Model file for the job. Use its own axes, mm. A direction names the side the tool comes from. Coordinates: 2 decimals unless noted, no trailing zeros. Order: outer loops, then holes, each group sorted by start corner. A loop starts at its lowest first (then second) coordinate and runs counter-clockwise, first axis right, second up. Notation, with made-up numbers: (-6.5, 30) -> (14.5, 30) arc R26 ccw to (14.5, 58) -> close; hole circle Ø3 at (-18, 80.25). An arc over 180 degrees is marked (long way). Return JSON: item names as keys, results as strings. Group by question number.
1) Pull direction Z, two halves, no side cores. Call faces 4 (the flat face through (-35, 2, 60)), 5 (the flat face through (-67.3, 118, 45.5)), 6 (the flat face through (-74, 121, 5)): +Z half, -Z half, draft (parallel to the pull), parting line (faces both ways), or undercut.
2) Cut at B-B (x = 58). Write the cut outline in (y, z), and give its area (3 significant figures).
3) Probe line 1 (Y direction, x = -75, z = -40); line 2 (X direction, y = 2.2, z = -52); line 3 (Y direction, x = -74.6, z = 12.5). List the from-to ranges inside material, lowest first.
4) Flat gauge pins, fed straight in: pin 1 (3.5 mm diameter, centred on x = -66, z = 46.9, fed in from +Y); pin 2 (10 mm diameter, centred on y = 49.5, z = -43.5, fed in from +X); pin 3 (2 mm diameter, centred on y = 117, z = 47.5, fed in from +X). Where does each tip first touch, or does it go through?
5) Cut at A-A (y = 113). Write the cut outline in (x, z), and give its area (3 significant figures).
6) Which spindle directions (+Z, -Z, +X, -X, +Y, -Y) get a long thin tool onto all of the face, cutting with end or side? Do faces 1 (the flat face through (-72, 67, 56.9)), 2 (the flat face through (-66, 116, 1)), 3 (the flat face through (-74, 57.418, 0)). Say none if no direction does.
from build123d import *

# Parameters (mm, degrees)
SKETCH1_W              = 154
SKETCH1_H              = 120
LARGE_WALL_OUTER_DEPTH = 3
SKETCH8_W              = 3
SKETCH8_H              = 120
SMALL_WALL_OUTER_DEPTH = 120.1
SKETCH10_W             = 113.8
SKETCH10_H             = 112.9
SMALL_WALL_INNER_DEPTH = 3
SKETCH14_W             = 113.8
SKETCH14_H             = 4
MOUNT_DEPTH            = 10
MOUNTING_NUTS_DEPTH    = 2
NUT_1_BOLT_HOLE_REACH  = 155.144
SKETCH18_R             = 1.5
NUT_2_BOLT_HOLE_REACH  = 155.144
SKETCH19_R             = 1.5
CONNECTOR_SLOTS_REACH  = 208.082
SKETCH23_R             = 1.5
SKETCH27_R             = 1.55
SKETCH27_R_2           = 1.5
PCB_MOUNT_HOLES_DEPTH  = 6
SKETCH28_R             = 1.5
BOLT_HOLE1_DEPTH       = 10
SKETCH29_R             = 1.5
BOLT_HOLE2_DEPTH       = 10
SKETCH30_R             = 1.5
BOLT_HOLES34_DEPTH     = 10


with BuildPart() as part:
    # Sketch1 → Large-Wall-Outer (new body)
    with BuildSketch(Plane(origin=(0, 0, 0), x_dir=(1, 0, 0), z_dir=(0, 1, 0))):
        Rectangle(SKETCH1_W, SKETCH1_H)
    extrude(amount=LARGE_WALL_OUTER_DEPTH)

    # Sketch8 → Small-Wall-Outer (add)
    with BuildSketch(Plane(origin=(0, 3, 0), x_dir=(1, 0, 0), z_dir=(0, 1, 0))):
        with Locations((-75.5, 0)):
            Rectangle(SKETCH8_W, SKETCH8_H)
    extrude(amount=SMALL_WALL_OUTER_DEPTH)

    # Sketch10 → Small-Wall-Inner (add)
    with BuildSketch(Plane(origin=(-74, 0, 0), x_dir=(0, 0, -1), z_dir=(1, 0, 0))):
        with Locations((0, 63.55)):
            Rectangle(SKETCH10_W, SKETCH10_H)
    extrude(amount=SMALL_WALL_INNER_DEPTH)

    # Sketch14 → Mount (add)
    with BuildSketch(Plane(origin=(-71, 0, 0), x_dir=(0, 0, -1), z_dir=(1, 0, 0))):
        with Locations((0, 118)):
            Rectangle(SKETCH14_W, SKETCH14_H)
    extrude(amount=MOUNT_DEPTH)

    # Sketch17 → Mounting-Nuts (cut)
    with BuildSketch(Plane.XZ.offset(-116)):
        Polygon((-66, 43.7), (-63.228718708, 45.3), (-63.228718708, 48.5), (-66, 50.1), (-68.771281292, 48.5), (-68.771281292, 45.3), align=None)
        Polygon((-66, -50.1), (-63.228718708, -48.5), (-63.228718708, -45.3), (-66, -43.7), (-68.771281292, -45.3), (-68.771281292, -48.5), align=None)
    extrude(amount=-MOUNTING_NUTS_DEPTH, mode=Mode.SUBTRACT)

    # Sketch18 → Nut-1-Bolt-Hole (cut, up to next)
    with BuildSketch(Plane.XZ.offset(-118), mode=Mode.PRIVATE) as nut_1_bolt_hole_sk1:
        with Locations(Location((-66, 46.9, 0), (0, 0, 270))):
            Circle(SKETCH18_R)
    nut_1_bolt_hole_tool1 = extrude(nut_1_bolt_hole_sk1.sketch, amount=-NUT_1_BOLT_HOLE_REACH, mode=Mode.PRIVATE) & part.part
    add(nut_1_bolt_hole_tool1.solids().sort_by_distance((-66, 118, 46.9))[0], mode=Mode.SUBTRACT)

    # Sketch19 → Nut-2-Bolt-Hole (cut, up to next)
    with BuildSketch(Plane.XZ.offset(-118), mode=Mode.PRIVATE) as nut_2_bolt_hole_sk1:
        with Locations(Location((-66, -46.9, 0), (0, 0, 270))):
            Circle(SKETCH19_R)
    nut_2_bolt_hole_tool1 = extrude(nut_2_bolt_hole_sk1.sketch, amount=-NUT_2_BOLT_HOLE_REACH, mode=Mode.PRIVATE) & part.part
    add(nut_2_bolt_hole_tool1.solids().sort_by_distance((-66, 118, -46.9))[0], mode=Mode.SUBTRACT)

    # Sketch23 → Connector-Slots (cut, up to next)
    with BuildSketch(Plane(origin=(-77, 0, 0), x_dir=(0, 0, -1), z_dir=(-1, 0, 0)), mode=Mode.PRIVATE) as connector_slots_sk1:
        with Locations(Location((-12.5, -63.05, 0), (0, 0, 180))):
            Circle(SKETCH23_R)
    connector_slots_tool1 = extrude(connector_slots_sk1.sketch, amount=-CONNECTOR_SLOTS_REACH, mode=Mode.PRIVATE) & part.part
    # Sketch23 → Connector-Slots (cut, up to next)
    with BuildSketch(Plane(origin=(-77, 0, 0), x_dir=(0, 0, -1), z_dir=(-1, 0, 0)), mode=Mode.PRIVATE) as connector_slots_sk2:
        with Locations(Location((12.5, -63.05, 0), (0, 0, 180))):
            Circle(SKETCH23_R)
    connector_slots_tool2 = extrude(connector_slots_sk2.sketch, amount=-CONNECTOR_SLOTS_REACH, mode=Mode.PRIVATE) & part.part
    # Sketch23 → Connector-Slots (cut, up to next)
    with BuildSketch(Plane(origin=(-77, 0, 0), x_dir=(0, 0, -1), z_dir=(-1, 0, 0)), mode=Mode.PRIVATE) as connector_slots_sk3:
        with Locations(Location((-23.52, -78.05, 0), (0, 0, 180))):
            Circle(SKETCH23_R)
    connector_slots_tool3 = extrude(connector_slots_sk3.sketch, amount=-CONNECTOR_SLOTS_REACH, mode=Mode.PRIVATE) & part.part
    # Sketch23 → Connector-Slots (cut, up to next)
    with BuildSketch(Plane(origin=(-77, 0, 0), x_dir=(0, 0, -1), z_dir=(-1, 0, 0)), mode=Mode.PRIVATE) as connector_slots_sk4:
        with Locations(Location((23.52, -78.05, 0), (0, 0, 180))):
            Circle(SKETCH23_R)
    connector_slots_tool4 = extrude(connector_slots_sk4.sketch, amount=-CONNECTOR_SLOTS_REACH, mode=Mode.PRIVATE) & part.part
    # Sketch23 → Connector-Slots (cut, up to next)
    with BuildSketch(Plane(origin=(-77, 0, 0), x_dir=(0, 0, -1), z_dir=(-1, 0, 0)), mode=Mode.PRIVATE) as connector_slots_sk5:
        with Locations(Location((-23.52, -48.05, 0), (0, 0, 180))):
            Circle(SKETCH23_R)
    connector_slots_tool5 = extrude(connector_slots_sk5.sketch, amount=-CONNECTOR_SLOTS_REACH, mode=Mode.PRIVATE) & part.part
    # Sketch23 → Connector-Slots (cut, up to next)
    with BuildSketch(Plane(origin=(-77, 0, 0), x_dir=(0, 0, -1), z_dir=(-1, 0, 0)), mode=Mode.PRIVATE) as connector_slots_sk6:
        with Locations(Location((23.52, -48.05, 0), (0, 0, 180))):
            Circle(SKETCH23_R)
    connector_slots_tool6 = extrude(connector_slots_sk6.sketch, amount=-CONNECTOR_SLOTS_REACH, mode=Mode.PRIVATE) & part.part
    # Sketch23 → Connector-Slots (cut, up to next)
    with BuildSketch(Plane(origin=(-77, 0, 0), x_dir=(0, 0, -1), z_dir=(-1, 0, 0)), mode=Mode.PRIVATE) as connector_slots_sk7:
        with BuildLine():
            Line((-6.891594987, -68.167891943), (6.891594987, -68.167891943))
            ThreePointArc((6.891594987, -68.167891943), (8.211781315, -67.670259427), (8.875, -66.425))
            Line((8.875, -66.425), (9.75, -59.675))
            ThreePointArc((9.75, -59.675), (9.268962471, -58.097705614), (7.766594987, -57.417891943))
            Line((7.766594987, -57.417891943), (-7.766594987, -57.417891943))
            ThreePointArc((-7.766594987, -57.417891943), (-9.268962471, -58.097705614), (-9.75, -59.675))
            Line((-9.75, -59.675), (-8.875, -66.425))
            ThreePointArc((-8.875, -66.425), (-8.211781315, -67.670259427), (-6.891594987, -68.167891943))
        make_face()
    connector_slots_tool7 = extrude(connector_slots_sk7.sketch, amount=-CONNECTOR_SLOTS_REACH, mode=Mode.PRIVATE) & part.part
    # Sketch23 → Connector-Slots (cut, up to next)
    with BuildSketch(Plane(origin=(-77, 0, 0), x_dir=(0, 0, -1), z_dir=(-1, 0, 0)), mode=Mode.PRIVATE) as connector_slots_sk8:
        with BuildLine():
            Line((-17.652212152, -83.096202025), (17.652212152, -83.096202025))
            ThreePointArc((17.652212152, -83.096202025), (18.944961945, -82.62224199), (19.625, -81.425))
            Line((19.625, -81.425), (20.75, -74.675))
            ThreePointArc((20.75, -74.675), (20.303252117, -73.053452233), (18.777212152, -72.346202025))
            Line((18.777212152, -72.346202025), (-18.777212152, -72.346202025))
            ThreePointArc((-18.777212152, -72.346202025), (-20.303252117, -73.053452233), (-20.75, -74.675))
            Line((-20.75, -74.675), (-19.625, -81.425))
            ThreePointArc((-19.625, -81.425), (-18.944961945, -82.62224199), (-17.652212152, -83.096202025))
        make_face()
    connector_slots_tool8 = extrude(connector_slots_sk8.sketch, amount=-CONNECTOR_SLOTS_REACH, mode=Mode.PRIVATE) & part.part
    # Sketch23 → Connector-Slots (cut, up to next)
    with BuildSketch(Plane(origin=(-77, 0, 0), x_dir=(0, 0, -1), z_dir=(-1, 0, 0)), mode=Mode.PRIVATE) as connector_slots_sk9:
        with BuildLine():
            Line((-17.652212152, -53.096202025), (17.652212152, -53.096202025))
            ThreePointArc((17.652212152, -53.096202025), (18.944961945, -52.62224199), (19.625, -51.425))
            Line((19.625, -51.425), (20.75, -44.675))
            ThreePointArc((20.75, -44.675), (20.303252117, -43.053452233), (18.777212152, -42.346202025))
            Line((18.777212152, -42.346202025), (-18.777212152, -42.346202025))
            ThreePointArc((-18.777212152, -42.346202025), (-20.303252117, -43.053452233), (-20.75, -44.675))
            Line((-20.75, -44.675), (-19.625, -51.425))
            ThreePointArc((-19.625, -51.425), (-18.944961945, -52.62224199), (-17.652212152, -53.096202025))
        make_face()
    connector_slots_tool9 = extrude(connector_slots_sk9.sketch, amount=-CONNECTOR_SLOTS_REACH, mode=Mode.PRIVATE) & part.part
    add(connector_slots_tool1.solids().sort_by_distance((-77, 63.05, 12.5))[0], mode=Mode.SUBTRACT)
    add(connector_slots_tool2.solids().sort_by_distance((-77, 63.05, -12.5))[0], mode=Mode.SUBTRACT)
    add(connector_slots_tool3.solids().sort_by_distance((-77, 78.05, 23.52))[0], mode=Mode.SUBTRACT)
    add(connector_slots_tool4.solids().sort_by_distance((-77, 78.05, -23.52))[0], mode=Mode.SUBTRACT)
    add(connector_slots_tool5.solids().sort_by_distance((-77, 48.05, 23.52))[0], mode=Mode.SUBTRACT)
    add(connector_slots_tool6.solids().sort_by_distance((-77, 48.05, -23.52))[0], mode=Mode.SUBTRACT)
    add(connector_slots_tool7.solids().sort_by_distance((-77, 62.681741, 0))[0], mode=Mode.SUBTRACT)
    add(connector_slots_tool8.solids().sort_by_distance((-77, 77.655881, 0))[0], mode=Mode.SUBTRACT)
    add(connector_slots_tool9.solids().sort_by_distance((-77, 47.655881, 0))[0], mode=Mode.SUBTRACT)

    # Sketch27 → PCB-Mount-Holes (cut)
    with BuildSketch(Plane.ZY.offset(77)):
        with Locations((-40, 23.05)):
            Circle(SKETCH27_R)
        with Locations((12.5, 63.05)):
            Circle(SKETCH27_R_2)
        with Locations((-12.5, 63.05)):
            Circle(SKETCH27_R_2)
        with Locations((40, 23.05)):
            Circle(SKETCH27_R)
        with Locations((40, 103.05)):
            Circle(SKETCH27_R)
        with Locations((-40, 103.05)):
            Circle(SKETCH27_R)
    extrude(amount=-PCB_MOUNT_HOLES_DEPTH, mode=Mode.SUBTRACT)

    # Sketch28 → bolt-hole1 (cut)
    with BuildSketch(Plane(origin=(0, 3, 0), x_dir=(1, 0, 0), z_dir=(0, 1, 0))):
        with Locations(Location((-59, -52, 0), (0, 0, 270))):
            Circle(SKETCH28_R)
    extrude(amount=-BOLT_HOLE1_DEPTH, mode=Mode.SUBTRACT)

    # Sketch29 → bolt-hole2 (cut)
    with BuildSketch(Plane(origin=(0, 0, 0), x_dir=(-1, 0, 0), z_dir=(0, -1, 0))):
        with Locations(Location((-41, -52, 0), (0, 0, 90))):
            Circle(SKETCH29_R)
    extrude(amount=-BOLT_HOLE2_DEPTH, mode=Mode.SUBTRACT)

    # Sketch30 → bolt-holes34 (cut)
    with BuildSketch(Plane.XZ):
        with Locations(Location((-59, -52, 0), (0, 0, 270))):
            Circle(SKETCH30_R)
        with Locations(Location((41, -52, 0), (0, 0, 270))):
            Circle(SKETCH30_R)
    extrude(amount=-BOLT_HOLES34_DEPTH, mode=Mode.SUBTRACT)


solid = part.part
Answers below:
{
 "1": {"face 4": "+Z half", "face 5": "undercut", "face 6": "draft"},
 "2": {"outline": "(0, -60) -> (3, -60) -> (3, 60) -> (0, 60) -> close", "area": "360 mm^2"},
 "3": {"line 1": "y = 0 to 21.5, 24.6 to 101.5, 104.6 to 123.1", "line 2": "x = -77 to -60.5, -57.5 to 39.5, 42.5 to 77", "line 3": "y = 0 to 42.35, 53.1 to 61.55, 64.55 to 72.35, 83.1 to 123.1"},
 "4": {"pin 1": "stops at y = 120", "pin 2": "stops at x = -71", "pin 3": "stops at x = -61"},
 "5": {"outline": "(-77, -60) -> (-74, -60) -> (-74, -56.9) -> (-71, -56.9) -> (-71, 56.9) -> (-74, 56.9) -> (-74, 60) -> (-77, 60) -> close", "area": "701 mm^2"},
 "6": {"face 1": "+Z, +X, +Y", "face 2": "+Z, -Z, +X", "face 3": "+X, -X"}
}
